Model file for the job. Use its own axes, mm. A direction names the side the tool comes from. Round coordinates to 2 decimals unless told otherwise and drop trailing zeros. Loops run counter-clockwise (first coordinate to the right, second up) from the corner with the lowest first, then second, coordinate; pieces in that order, holes last. Notation, with made-up numbers: M 31,48 L 35,48 A21 cw 35,79 Z; hole C -1,6 d9. An arc over 180 degrees is marked long. Answer in a Markdown table with one row per item.
from build123d import *

# Parameters (mm, degrees)
BOSS_EXTRUDE1_DEPTH      = 3.175
BOSS_EXTRUDE1_DEPTH_BACK = 3.175
SKETCH1_R                = 3.1
SKETCH1_R_2              = 2.6


with BuildPart() as part:
    # Sketch1 → Boss-Extrude1 (new, two sides: drawn at the far end of the back side and taken through both)
    with BuildSketch(Plane(origin=(0, 0, 0), x_dir=(1, 0, 0), z_dir=(0, 1, 0)).offset(-BOSS_EXTRUDE1_DEPTH_BACK)):
        Polygon((-12.5, 0), (-12.5, -10), (12.5, -10), (12.5, 0), (12.5, 20), (-90, 20), (-90, 0), align=None)
        with Locations(Location((0, 0, 0), (0, 0, 270))):
            Circle(SKETCH1_R, mode=Mode.SUBTRACT)
        with Locations(Location((-40, 10, 0), (0, 0, 270))):
            Circle(SKETCH1_R_2, mode=Mode.SUBTRACT)
        with Locations(Location((-80, 10, 0), (0, 0, 270))):
            Circle(SKETCH1_R_2, mode=Mode.SUBTRACT)
    extrude(amount=BOSS_EXTRUDE1_DEPTH + BOSS_EXTRUDE1_DEPTH_BACK)


solid = part.part
1. Tool access for faces 5 (the flat face through (-52, 0, 0)), 6 (the flat face through (-39, 3.175, -5)): list every direction of +Z, -Z, +X, -X, +Y, -Y with a clear straight run to the whole face (end or side of a thin tool).
Verdict:
| item | result |
|---|---|
| face 5 | +Z, -X, +Y, -Y |
| face 6 | +Z, -Z, +X, -X, +Y |
2. Saw through at C-C (x = -80). Write the cut outline in (y, z) (3 decimals), and give its area (3 significant figures).
Verdict:
| item | result |
|---|---|
| outline | M -3.175,-20 L 3.175,-20 L 3.175,-12.6 L -3.175,-12.6 Z; M -3.175,-7.4 L 3.175,-7.4 L 3.175,0 L -3.175,0 Z |
| area | 94.0 mm² |
3. Wall check: probe 1 along X at (y, z) = (2.75, -12); probe 2 along X at (y, z) = (-1, -11.5); probe 3 along Z at (x, y) = (-13.5, -1.25). Give the ranges that are in metal, low to high.
Verdict:
| item | result |
|---|---|
| probe 1 | x = -90 to -81.66, -78.34 to -41.66, -38.34 to 12.5 |
| probe 2 | x = -90 to -82.12, -77.88 to -42.12, -37.88 to 12.5 |
| probe 3 | z = -20 to 0 |
4. Saw through at D-D (z = -1.5). Write the cut outline in (x, y) (3 decimals), and give its area (3 significant figures).
Verdict:
| item | result |
|---|---|
| outline | M -90,-3.175 L -2.713,-3.175 L -2.713,3.175 L -90,3.175 Z; M 2.713,-3.175 L 12.5,-3.175 L 12.5,3.175 L 2.713,3.175 Z |
| area | 616 mm² |
5. Saw through at A-A (z = -10). Write the cut outline in (x, y) (3 decimals), and give its area (3 significant figures).
Verdict:
| item | result |
|---|---|
| outline | M -90,-3.175 L -82.6,-3.175 L -82.6,3.175 L -90,3.175 Z; M -77.4,-3.175 L -42.6,-3.175 L -42.6,3.175 L -77.4,3.175 Z; M -37.4,-3.175 L 12.5,-3.175 L 12.5,3.175 L -37.4,3.175 Z |
| area | 585 mm² |
6. Saw through at B-B (y = 0.5). Write the cut outline in (x, z), and give its area (3 significant figures).
Verdict:
| item | result |
|---|---|
| outline | M -90,-20 L 12.5,-20 L 12.5,10 L -12.5,10 L -12.5,0 L -90,0 Z; hole C -80,-10 d5.2; hole C -40,-10 d5.2; hole C 0,0 d6.2 |
| area | 2,230 mm² |
7. Mould opens along Z. For faces 1 (the flat face through (-38, 0, -20)), 2 (the cylindrical face through (-77.422, -0.044, -10.338)), 3 (the cylindrical face through (-42.307, -0.044, -8.8)), 4 (the flat face through (-12.5, 0, 5)) say: +Z half, -Z half, draft (parallel to the pull), parting line (faces both ways), or undercut.
Verdict:
| item | result |
|---|---|
| face 1 | -Z half |
| face 2 | undercut |
| face 3 | undercut |
| face 4 | draft |
